from build123d import *

# Parameters (mm, degrees)
CROQUIS1_W              = 160
CROQUIS1_H              = 160
CROQUIS1_W_2            = 150
CROQUIS1_H_2            = 150
SALIENTE_EXTRUIR1_DEPTH = 5
CROQUIS2_W              = 150
CROQUIS2_H              = 150
CROQUIS2_W_2            = 98
CROQUIS2_H_2            = 98
SALIENTE_EXTRUIR2_DEPTH = 1
CROQUIS3_W              = 102
CROQUIS3_H              = 102
CROQUIS3_W_2            = 100
CROQUIS3_H_2            = 100
CORTAR_EXTRUIR1_DEPTH   = 0.3


with BuildPart() as part:
    # Croquis1 → Saliente-Extruir1 (new body)
    with BuildSketch(Plane(origin=(0, 0, 0), x_dir=(1, 0, 0), z_dir=(0, 1, 0))):
        with Locations((75, 75)):
            Rectangle(CROQUIS1_W, CROQUIS1_H)
        with Locations((75, 75)):
            Rectangle(CROQUIS1_W_2, CROQUIS1_H_2, mode=Mode.SUBTRACT)
    extrude(amount=SALIENTE_EXTRUIR1_DEPTH)

    # Croquis2 → Saliente-Extruir2 (add)
    with BuildSketch(Plane(origin=(0, 5, 0), x_dir=(1, 0, 0), z_dir=(0, 1, 0))):
        with Locations((75, 75)):
            Rectangle(CROQUIS2_W, CROQUIS2_H)
        with Locations((75, 75)):
            Rectangle(CROQUIS2_W_2, CROQUIS2_H_2, mode=Mode.SUBTRACT)
    extrude(amount=-SALIENTE_EXTRUIR2_DEPTH)

    # Croquis3 → Cortar-Extruir1 (cut)
    with BuildSketch(Plane(origin=(0, 5, 0), x_dir=(1, 0, 0), z_dir=(0, 1, 0))):
        with Locations((75, 75)):
            Rectangle(CROQUIS3_W, CROQUIS3_H)
        with Locations((75, 75)):
            Rectangle(CROQUIS3_W_2, CROQUIS3_H_2, mode=Mode.SUBTRACT)
    extrude(amount=-CORTAR_EXTRUIR1_DEPTH, mode=Mode.SUBTRACT)


solid = part.part
For this review, take the finished solid that the model builds, in its own axes (mm). A direction names the side the tool comes from. Round coordinates to 2 decimals unless told otherwise and drop trailing zeros. Write each loop counter-clockwise with the first axis right and the second up, starting at its lowest first coordinate (ties: lowest second). Pieces come first, ordered by that corner, then holes. Notation, with made-up numbers: (34, 21.5) - (69, 21.5) arc R15 ccw to (69, 34.5) - close; hole circle Ø6 at (-11.5, 77.25). An arc over 180 degrees is marked (long way). Use a Markdown table: item, result.
Q1. We need section D-D (x = 143). Give the boundary of the cut face in (y, z), plus the area to 3 significant figures.
Derived:
| item | result |
|---|---|
| outline | (0, -155) - (5, -155) - (5, 5) - (0, 5) - (0, 0) - (4, 0) - (4, -150) - (0, -150) - close |
| area | 200 mm2 |
Q2. We need section B-B (y = 0.9). Give the boundary of the cut face in (x, z).
Derived:
| item | result |
|---|---|
| outline | (-5, -155) - (155, -155) - (155, 5) - (-5, 5) - close; hole (0, -150) - (150, -150) - (150, 0) - (0, 0) - close |
Q3. Wall thickness on line 1 along Z through (x, y) = (74, 4.8); line 2 along Z through (x, y) = (95, 0.4); line 3 along X through (y, z) = (2.1, -73.5): over which ranges is each line inside the solid? List them lowest first.
Derived:
| item | result |
|---|---|
| line 1 | z = -155 to -126, -125 to -124, -26 to -25, -24 to 5 |
| line 2 | z = -155 to -150, 0 to 5 |
| line 3 | x = -5 to 0, 150 to 155 |
Q4. Machinability: for faces 4 (the flat face through (150, 2, -74)), 5 (the flat face through (-5, 2, -74)), which of the approach directions +Z, -Z, +X, -X, +Y, -Y give a long, thin tool a straight path to every point of the face, cutting with its end or side? Answer none if there is none.
Derived:
| item | result |
|---|---|
| face 4 | -Y |
| face 5 | +Z, -Z, -X, +Y, -Y |
Q5. We need section C-C (z = -70). Give the boundary of the cut face in (x, y).
Derived:
| item | result |
|---|---|
| outline | (-5, 0) - (0, 0) - (0, 4) - (26, 4) - (26, 5) - (25, 5) - (25, 4.7) - (24, 4.7) - (24, 5) - (-5, 5) - close; (124, 4) - (150, 4) - (150, 0) - (155, 0) - (155, 5) - (126, 5) - (126, 4.7) - (125, 4.7) - (125, 5) - (124, 5) - close |
Q6. The part is to be moulded in two halves that separate along X. For faces 1 (the flat face through (0, 2, -74)), 2 (the flat face through (69, 0, 2)), 3 (the flat face through (155, 2, -74)), say which applies: pulls with the +X half, pulls with the -X half, needs draft (parallel to the pull), parting line crosses it, or undercut.
Derived:
| item | result |
|---|---|
| face 1 | undercut |
| face 2 | needs draft |
| face 3 | pulls with the +X half |
Q7. We need section A-A (x = 49.5). Give the boundary of the cut face in (y, z), plus the area to 3 significant figures.
Derived:
| item | result |
|---|---|
| outline | (0, -155) - (5, -155) - (5, -126) - (4.7, -126) - (4.7, -125) - (5, -125) - (5, -124) - (4, -124) - (4, -150) - (0, -150) - close; (0, 0) - (4, 0) - (4, -26) - (5, -26) - (5, -25) - (4.7, -25) - (4.7, -24) - (5, -24) - (5, 5) - (0, 5) - close |
| area | 101 mm2 |
